Source: three-view drawing plus pictorial views. Frame: mm from the lowest corner of the part. Coordinates: 2 decimals unless noted, no trailing zeros. Loops run counter-clockwise (first coordinate to the right, second up) from the corner with the lowest first, then second, coordinate; pieces in that order, holes last. Notation, with made-up numbers: (-11.5, 19) - (2.5, 19) arc R30 cw to (2.5, 48) - close; hole circle Ø3 at (68, -5). An arc over 180 degrees is marked (long way). Return JSON: item names as keys, results as strings.
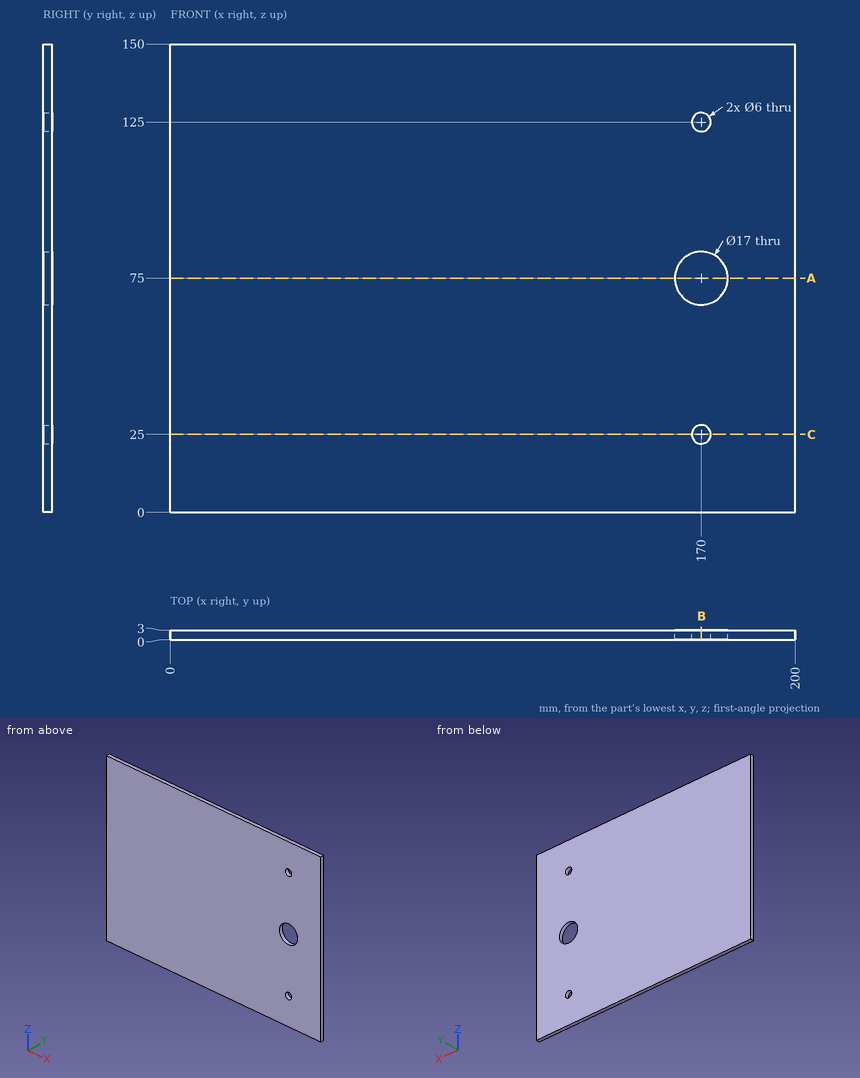
Item 1: First-contact query: pin 1 Ø3.5 at (x, z) = (170, 25) entering from -Y. Flat tip, straight axial feed; report the tip coordinate or a pass-through.
Worked out:
{"pin 1": "through"}
Item 2: Ray query, probe 1 along Z at (x, y) = (170, 1.25); probe 2 along Z at (x, y) = (172, 1.1); probe 3 along X at (y, z) = (0.95, 72). Return the intervals inside material, ascending. Write a range as from..to.
Worked out:
{"probe 1": "0..22, 28..66.5, 83.5..122, 128..150", "probe 2": "0..22.76, 27.24..66.74, 83.26..122.76, 127.24..150", "probe 3": "0..162.05, 177.95..200"}
Item 3: Section query C-C, the plane z = 25. Return loops of the section in (x, y).
Worked out:
{"outline": "(0, 0) - (167, 0) - (167, 3) - (0, 3) - close; (173, 0) - (200, 0) - (200, 3) - (173, 3) - close"}
Item 4: Section query A-A, the plane z = 75. Return loops of the section in (x, y), and give its area (3 significant figures).
Worked out:
{"outline": "(0, 0) - (161.5, 0) - (161.5, 3) - (0, 3) - close; (178.5, 0) - (200, 0) - (200, 3) - (178.5, 3) - close", "area": "549 mm^2"}
Item 5: Section query B-B, the plane x = 170. Return loops of the section in (y, z).
Worked out:
{"outline": "(0, 0) - (3, 0) - (3, 22) - (0, 22) - close; (0, 28) - (3, 28) - (3, 66.5) - (0, 66.5) - close; (0, 83.5) - (3, 83.5) - (3, 122) - (0, 122) - close; (0, 128) - (3, 128) - (3, 150) - (0, 150) - close"}
